from build123d import *

# Parameters (mm, degrees)
SKETCH_1_W      = 20
SKETCH_1_H      = 20
EXTRUDE_1_DEPTH = 2
SKETCH_2_W      = 20
SKETCH_2_H      = 10
EXTRUDE_3_DEPTH = 2
SKETCH_4_W      = 20
SKETCH_4_H      = 10
EXTRUDE_4_DEPTH = 2
SKETCH_5_W      = 10
SKETCH_5_H      = 24
EXTRUDE_5_DEPTH = 2
SKETCH_6_W      = 10
SKETCH_6_H      = 24
EXTRUDE_6_DEPTH = 2


with BuildPart() as part:
    # 草图1 → 凸台-拉伸1 (new body)
    with BuildSketch(Plane.XY):
        Rectangle(SKETCH_1_W, SKETCH_1_H)
    extrude(amount=EXTRUDE_1_DEPTH)

    # 草图2 → 凸台-拉伸3 (add)
    with BuildSketch(Plane.XZ.offset(10)):
        with Locations((0, 5)):
            Rectangle(SKETCH_2_W, SKETCH_2_H)
    extrude(amount=EXTRUDE_3_DEPTH)

    # 草图4 → 凸台-拉伸4 (add)
    with BuildSketch(Plane(origin=(0, 10, 0), x_dir=(1, 0, 0), z_dir=(0, 1, 0))):
        with Locations((0, -5)):
            Rectangle(SKETCH_4_W, SKETCH_4_H)
    extrude(amount=EXTRUDE_4_DEPTH)

    # 草图5 → 凸台-拉伸5 (add)
    with BuildSketch(Plane(origin=(10, 0, 0), x_dir=(0, 0, -1), z_dir=(1, 0, 0))):
        with Locations((-5, 0)):
            Rectangle(SKETCH_5_W, SKETCH_5_H)
    extrude(amount=EXTRUDE_5_DEPTH)

    # 草图6 → 凸台-拉伸6 (add)
    with BuildSketch(Plane.ZY.offset(10)):
        with Locations((5, 0)):
            Rectangle(SKETCH_6_W, SKETCH_6_H)
    extrude(amount=EXTRUDE_6_DEPTH)


solid = part.part
The listing builds one solid part. Answer for the finished solid, in the listing's coordinates (mm). A direction names the side the tool comes from. Coordinates: 2 decimals unless noted, no trailing zeros. Order: outer loops, then holes, each group sorted by start corner. A loop starts at its lowest first (then second) coordinate and runs counter-clockwise, first axis right, second up. Notation, with made-up numbers: (-24.5, 20.5) -> (15.5, 20.5) arc R15 cw to (15.5, 46.5) -> close; hole circle Ø6 at (-32.5, -31). An arc over 180 degrees is marked (long way). Answer in a Markdown table with one row per item. Add a question column.
Item 1: Which of the six approach directions +Z, -Z, +X, -X, +Y, -Y give full straight-line access (tool end or side, diameter ignored) to faces 1 (the face through (-12, 0, 5)), 2 (the face through (0, 0, 2))?
Item 2: Find the intervals of material crossed by L1, parallel to Y at x = -5.75, z = 2.5; L2, parallel to Z at x = 9.75, y = -0.5, in increasing order. Write a range as from..to.
Item 3: Determine the mould class of faces 3 (the face through (0, 0, 0)), 4 (the face through (0, -12, 5)), 5 (the face through (0, 10, 6)), 6 (the face through (0, 12, 5)) for opening direction Y: +Y half, -Y half, draft (parallel to the pull), parting line (faces both ways), or undercut.
Item 4: This flat-tipped pin is pushed along its axis until it touches: P1, Ø6, axis at x = -4, y = 1.5, coming from the +Z side. Where does it stop, or does it pass through?
Item 5: Find section B-B (z = 6). Write down the section's boundary in (x, y), then the cut area to 3 significant figures.
Item 6: Find section A-A (x = -1.75). Write down the section's boundary in (y, z), then the cut area to 3 significant figures.
Result set:
| question | item | result |
|---|---|---|
| 1 | face 1 | +Z, -Z, -X, +Y, -Y |
| 1 | face 2 | +Z |
| 2 | L1 | y = -12..-10, 10..12 |
| 2 | L2 | z = 0..2 |
| 3 | face 3 | draft |
| 3 | face 4 | -Y half |
| 3 | face 5 | undercut |
| 3 | face 6 | +Y half |
| 4 | P1 | stops at z = 2 |
| 5 | outline | (-12, -12) -> (12, -12) -> (12, 12) -> (-12, 12) -> close; hole (-10, -10) -> (10, -10) -> (10, 10) -> (-10, 10) -> close |
| 5 | area | 176 mm² |
| 6 | outline | (-12, 0) -> (12, 0) -> (12, 10) -> (10, 10) -> (10, 2) -> (-10, 2) -> (-10, 10) -> (-12, 10) -> close |
| 6 | area | 80.0 mm² |
